Part model, mm, in its own coordinate system. A direction names the side the tool comes from. Give positions to 0.01 mm unless a question says otherwise; leave off trailing zeros. Loops run counter-clockwise (first coordinate to the right, second up) from the corner with the lowest first, then second, coordinate; pieces in that order, holes last. Notation, with made-up numbers: M 84,14 L 125,14 A12 ccw 125,25 Z; hole C 54,-6 d2. An arc over 180 degrees is marked long. Answer in a Markdown table with one row per item.
from build123d import *

# Parameters (mm, degrees)
SKETCH1_W                            = 120
SKETCH1_H                            = 50
BOSS_EXTRUDE1_DEPTH                  = 5
SKETCH2_W                            = 5
SKETCH2_H                            = 50
BOSS_EXTRUDE2_DEPTH                  = 10
F_3_5_3_5_DIAMETER_HOLE1_D           = 3.5
F_3_5_3_5_DIAMETER_HOLE1_CSINK_D     = 3.55
F_3_5_3_5_DIAMETER_HOLE1_CSINK_ANGLE = 90


with BuildPart() as part:
    # Sketch1 → Boss-Extrude1 (new body)
    with BuildSketch(Plane(origin=(0, 0, 0), x_dir=(1, 0, 0), z_dir=(0, 1, 0))):
        Rectangle(SKETCH1_W, SKETCH1_H)
    extrude(amount=BOSS_EXTRUDE1_DEPTH)

    # Sketch2 → Boss-Extrude2 (add)
    with BuildSketch(Plane(origin=(0, 5, 0), x_dir=(1, 0, 0), z_dir=(0, 1, 0))):
        with Locations((-57.5, 0)):
            Rectangle(SKETCH2_W, SKETCH2_H)
        with Locations((57.5, 0)):
            Rectangle(SKETCH2_W, SKETCH2_H)
    extrude(amount=BOSS_EXTRUDE2_DEPTH)

    # Ø3.5 (3.5) Diameter Hole1 (through all)
    with Locations(Plane(origin=(60, 0, 0), x_dir=(0, 0, -1), z_dir=(1, 0, 0))):
        with Locations((-20, 10), (20, 10)):
            CounterSinkHole(F_3_5_3_5_DIAMETER_HOLE1_D / 2, F_3_5_3_5_DIAMETER_HOLE1_CSINK_D / 2, counter_sink_angle=F_3_5_3_5_DIAMETER_HOLE1_CSINK_ANGLE)


solid = part.part
(1) Saw through at D-D (x = 0). Write the cut outline in (y, z), plus the area to 3 significant figures.
Recorded:
| item | result |
|---|---|
| outline | M 0,-25 L 5,-25 L 5,25 L 0,25 Z |
| area | 250 mm^2 |
(2) Pin check, flat tips, straight feed: pin 1 Ø3 at (y, z) = (10, 20) entering from +X; pin 2 Ø12 at (x, z) = (-40, 2.5) entering from +Y; pin 3 Ø4.5 at (y, z) = (10, -20) entering from -X. Stop position of each tip, or through.
Recorded:
| item | result |
|---|---|
| pin 1 | passes through |
| pin 2 | stops at y = 5 |
| pin 3 | stops at x = -60 |
(3) Which spindle directions (+Z, -Z, +X, -X, +Y, -Y) get a long thin tool onto all of the face, cutting with end or side? Do faces 1 (the face through (-57.54, 11.18, -21.29)), 2 (the face through (55, 10, 0)). Say none if no direction does.
Recorded:
| item | result |
|---|---|
| face 1 | +X, -X |
| face 2 | +Z, -Z, +Y |
(4) Saw through at A-A (z = 20). Write the cut outline in (x, y) (3 decimals).
Recorded:
| item | result |
|---|---|
| outline | M -60,0 L 60,0 L 60,8.225 L 59.975,8.25 L 55,8.25 L 55,5 L -55,5 L -55,8.25 L -60,8.25 Z; M -60,11.75 L -55,11.75 L -55,15 L -60,15 Z; M 55,11.75 L 59.975,11.75 L 60,11.775 L 60,15 L 55,15 Z |
(5) Saw through at B-B (y = 10). Write the cut outline in (x, z) (3 decimals).
Recorded:
| item | result |
|---|---|
| outline | M -60,-25 L -55,-25 L -55,-21.75 L -60,-21.75 Z; M -60,-18.25 L -55,-18.25 L -55,18.25 L -60,18.25 Z; M -60,21.75 L -55,21.75 L -55,25 L -60,25 Z; M 55,-25 L 60,-25 L 60,-21.775 L 59.975,-21.75 L 55,-21.75 Z; M 55,-18.25 L 59.975,-18.25 L 60,-18.225 L 60,18.225 L 59.975,18.25 L 55,18.25 Z; M 55,21.75 L 59.975,21.75 L 60,21.775 L 60,25 L 55,25 Z |
(6) Drill centre lines: line 1 along Z through (x, y) = (58.8, 10); line 2 along Y through (x, z) = (56.15, 20); line 3 along X through (y, z) = (9.5, 1). Where is each one in solid material? Low to high.
Recorded:
| item | result |
|---|---|
| line 1 | z = -25 to -21.75, -18.25 to 18.25, 21.75 to 25 |
| line 2 | y = 0 to 8.25, 11.75 to 15 |
| line 3 | x = -60 to -55, 55 to 60 |
(7) Saw through at C-C (z = 7). Write the cut outline in (x, y), plus the area to 3 significant figures.
Recorded:
| item | result |
|---|---|
| outline | M -60,0 L 60,0 L 60,15 L 55,15 L 55,5 L -55,5 L -55,15 L -60,15 Z |
| area | 700 mm^2 |
(8) Pull direction Y, two halves, no side cores. Call faces 3 (the face through (-1, 0, 0)), 4 (the face through (57.45, 11.18, 18.71)), 5 (the face through (0, 4, 25)), 6 (the face through (-57.54, 11.18, 18.71)): +Y half, -Y half, draft (parallel to the pull), parting line (faces both ways), or undercut.
Recorded:
| item | result |
|---|---|
| face 3 | -Y half |
| face 4 | undercut |
| face 5 | draft |
| face 6 | undercut |
